Autodesk Inventor part; units mm, degrees
ref_plane "YZ Plane" through (0, 0, 0) normal (1, 0, 0) x (0, 1, 0)
ref_plane "XZ Plane" through (0, 0, 0) normal (0, 1, 0) x (-1, 0, 0)
ref_plane "XY Plane" through (0, 0, 0) normal (0, 0, 1) x (1, 0, 0)
sketch "Sketch1" plane through (0, 0, 0) normal (1, 0, 0) x (0, 1, 0)
  line L0 (-50, 489.5) -> (50, 489.5)
  line L1 (50, 489.5) -> (50, -489.5)
  line L2 (50, -489.5) -> (-50, -489.5)
  line L3 (-50, -489.5) -> (-50, 489.5)
  line L4 (-50, 489.5) -> (50, -489.5) construction
  line L5 (50, 489.5) -> (-50, -489.5) construction
  point P0 (0, 0)
  dimension "d0" = 979
  dimension "d1" = 100
extrude "Extrusion1" add sketch "Sketch1" along normal blind 5
sketch "Sketch2" plane through (5, 0, 0) normal (1, 0, 0) x (0, 0, -1)
  circle A0 centre (-270.411, -31.452) radius 12.25
  line L0 (-489.5, -50) -> (489.5, -50)
  line L1 (-489.5, 50) -> (-489.5, -50)
  circle A1 centre (274.562, -31.452) radius 12.25
  line L2 (489.5, -50) -> (489.5, 50)
  point P0 (0, 0)
  dimension "d4" = 24.5
  dimension "d5" = 18.548
  dimension "d8" = 219.089
  dimension "d18" = 214.938
  dimension "d19" = 24.5
  dimension "d20" = 18.548
extrude "Extrusion2" cut sketch "Sketch2" against normal through all
sketch "Sketch6" plane through (5, 0, 0) normal (1, 0, 0) x (0, 0, -1)
  circle A0 centre (274.5619, -31.452) radius 16.3
  circle A1 centre (212.908, -30) radius 2.75
  circle A2 centre (-124.274, -40) radius 2.75
  circle A3 centre (-164.274, 40) radius 2.75
  circle A4 centre (313.651, 40.5) radius 2.75
  circle A5 centre (433.651, 40.5) radius 2.75
  circle A6 centre (-309.5, 40.5) radius 2.75
  circle A7 centre (-85, -34.5) radius 2.75
  circle A8 centre (-186, 30) radius 2.75
  circle A9 centre (92.5, -34.5) radius 2.75
  circle A10 centre (185.908, -30) radius 2.75
  circle A11 centre (185.908, 30) radius 2.75
  circle A12 centre (92.5, 34.5) radius 2.75
  circle A13 centre (-186, -30) radius 2.75
  circle A14 centre (-85, 34.5) radius 2.75
  circle A15 centre (-429.5, 40.5) radius 2.75
  circle A16 centre (-369.5, 40.5) radius 2.75
  circle A17 centre (373.651, 40.5) radius 2.75
  circle A18 centre (-124.274, 40) radius 2.75
  circle A19 centre (-154.274, -40) radius 2.75
  circle A20 centre (212.908, 30) radius 2.75
  circle A21 centre (148.424, 0) radius 9.8
  circle A22 centre (-61.972, 12.7) radius 2.25
  circle A23 centre (-87.372, 12.7) radius 2.25
  circle A24 centre (-87.372, -12.7) radius 2.25
  circle A25 centre (-61.972, -12.7) radius 2.25
  line L0 (-19.5, -25) -> (-19.5, 25)
  line L1 (-19.5, 25) -> (110.5, 25)
  line L2 (110.5, 25) -> (110.5, -25)
  line L3 (110.5, -25) -> (-19.5, -25)
  circle A26 centre (-144.273, 0) radius 30
  arc A27 (-360.3076, -42.4652) -> (-351.3744, -41.3708) centre (-355.841, -41.918) ccw
  arc A28 (-360.9797, -31.4275) -> (-360.3076, -42.4652) centre (-270.411, -31.452) ccw
  arc A29 (-351.9797, -31.4299) -> (-360.9797, -31.4275) centre (-356.4797, -31.4287) ccw
  arc A30 (-351.9797, -31.4299) -> (-351.3744, -41.3708) centre (-270.411, -31.452) ccw
  circle A31 centre (-270.411, -31.452) radius 16.3
  line L4 (-469.5, 50) -> (-469.5, -50)
  line L5 (-469.5, -50) -> (469.5, -50)
  line L6 (469.5, 50) -> (469.5, -50)
  line L7 (-469.5, 50) -> (469.5, 50)
  circle A32 centre (128.424, -40) radius 2.75
  circle A33 centre (128.424, 40) radius 2.75
  circle A34 centre (168.424, 40) radius 2.75
  circle A35 centre (158.424, -40) radius 2.75
  point P0 (0, 0)
extrude "Extrusion4" cut sketch "Sketch6" against normal blind 10 contours A1 | A4 | A5 | A6 | A7 | A8 | A9 | A10 | A11 | A12 | A13 | A14 | A15 | A16 | A17 | A20
equation "\"d20\" = d5"
properties part number "Bumper Plate" material "Aluminum 6061"
Can you work these out from the model? Positions are in its coordinate system, mm. Round coordinates to 2 decimals unless told otherwise and drop trailing zeros. One line per question, with ' | ' between items. Start each with the question number.
1) I'm going to push a flat-ended pin straight in: P1, Ø14.5, axis at y = -31.452, z = -274.562, coming from the +X side. Where does the tip first touch, or does it pass through?
2) I need wall thicknesses on line 1 (Y direction, x = 3.9, z = -92.5); line 2 (Y direction, x = 2.2, z = 369.5); line 3 (Y direction, x = 1.45, z = -94.5). Which ranges of each line are inside material? Lowest first, please. Write a range as [from, to].
3) If we mould it in two halves opening along Z, with no side actions, what happens to faces 1 (the cylindrical face through (2.54, -36.14, -285.88)), 2 (the cylindrical face through (2.54, -38.91, 280.13)), 3 (the flat face through (0, -1, 7))? For each: released by +Z, released by -Z, zero draft, split by the parting line, or undercut.
Return value:
1) P1: passes through
2) line 1: y = [-50, -37.25], [-31.75, 31.75], [37.25, 50] | line 2: y = [-50, 37.75], [43.25, 50] | line 3: y = [-50, -36.39], [-32.61, 32.61], [36.39, 50]
3) face 1: undercut | face 2: undercut | face 3: zero draft
